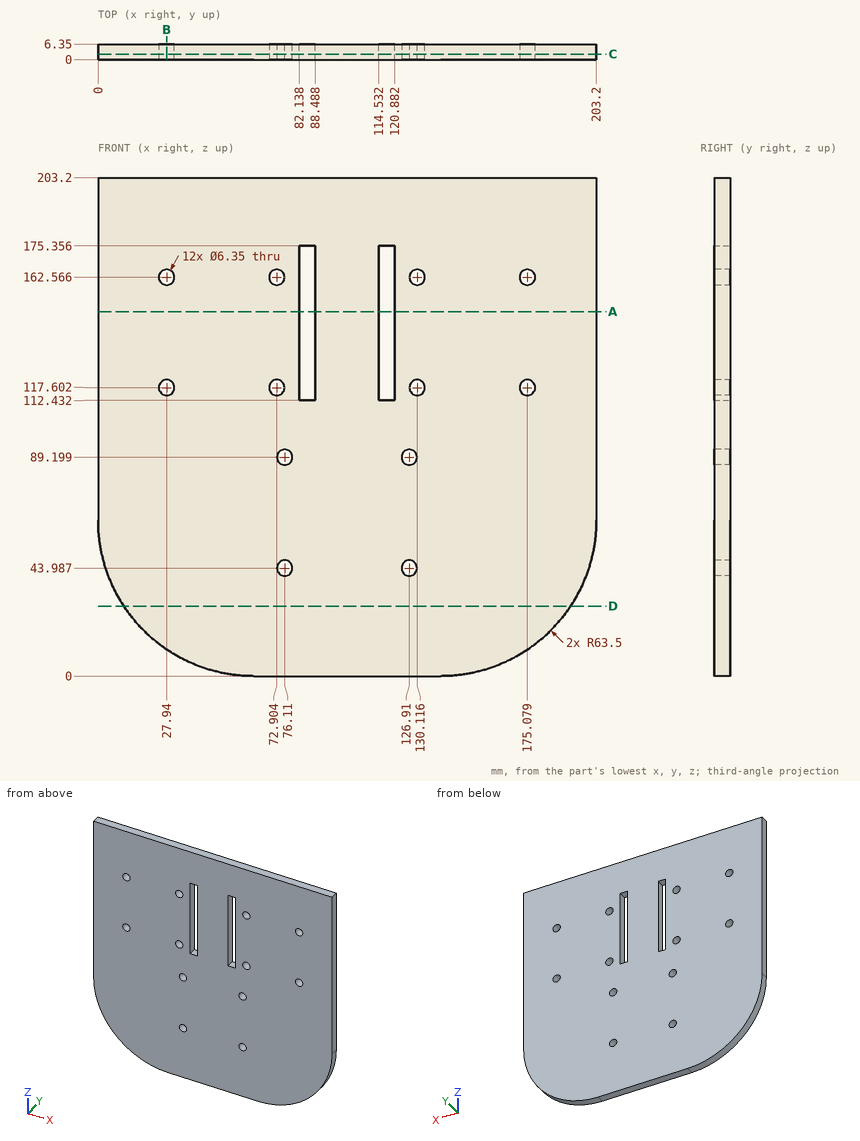
Geometry: see drawing. Coordinates: mm, zero at the bounding-box minimum. Coordinates: 2 decimals unless noted, no trailing zeros. Loops run counter-clockwise (first coordinate to the right, second up) from the corner with the lowest first, then second, coordinate; pieces in that order, holes last. Notation, with made-up numbers: (40, 38) - (44, 38) arc R24 cw to (44, 77) - close; hole circle Ø9 at (54.5, 85). An arc over 180 degrees is marked (long way). Answer in a Markdown table with one row per item.
(1) Cut plane B-B on x = 27.94. Output: boundary loops of the cut face in (y, z), plus the area to 3 significant figures.
Model answer:
| item | result |
|---|---|
| outline | (0, 10.89) - (6.35, 10.89) - (6.35, 114.43) - (0, 114.43) - close; (0, 120.78) - (6.35, 120.78) - (6.35, 159.39) - (0, 159.39) - close; (0, 165.74) - (6.35, 165.74) - (6.35, 203.2) - (0, 203.2) - close |
| area | 1,140 mm² |
(2) Cut plane C-C on y = 2.25. Count the separate pieces of the cut face and the enclosed holes in it, plus the area to 3 significant figures.
Model answer:
| item | result |
|---|---|
| separate pieces | 1 |
| enclosed holes | 14 |
| area | 38,400 mm² |
(3) Cut plane A-A on z = 148.5. Output: boundary loops of the cut face in (x, y).
Model answer:
| item | result |
|---|---|
| outline | (0, 0) - (82.14, 0) - (82.14, 6.35) - (0, 6.35) - close; (88.49, 0) - (114.53, 0) - (114.53, 6.35) - (88.49, 6.35) - close; (120.88, 0) - (203.2, 0) - (203.2, 6.35) - (120.88, 6.35) - close |
(4) Material intervals for L1, parallel to X at y = 6, z = 143; L2, parallel to Z at x = 76.5, y = 5.75; L3, parallel to Z at x = 74, y = 5.75 (1 decimal), sorted ascending. Write a range as from..to.
Model answer:
| item | result |
|---|---|
| L1 | x = 0..82.14, 88.49..114.53, 120.88..203.2 |
| L2 | z = 0..40.84, 47.14..86.05, 92.35..203.2 |
| L3 | z = 0..41.6, 46.4..86.8, 91.6..114.6, 120.6..159.6, 165.5..203.2 |
(5) Cut plane D-D on z = 28.5. Output: boundary loops of the cut face in (x, y).
Model answer:
| item | result |
|---|---|
| outline | (10.52, 0) - (192.68, 0) - (192.68, 6.35) - (10.52, 6.35) - close |
